Design review of the part built by this model. Coordinates are the model's own, in mm. Face numbers are marked on the shaded views. A direction names the side the tool comes from. Coordinates: 2 decimals unless noted, no trailing zeros. Loops run counter-clockwise (first coordinate to the right, second up) from the corner with the lowest first, then second, coordinate; pieces in that order, holes last. Notation, with made-up numbers: (-0.5, 78.5) - (16.5, 78.5) arc R23 cw to (16.5, 116.5) - close; hole circle Ø11 at (73, 28). An arc over 180 degrees is marked (long way). Use one line per item in the form item = value. Start each with the question number.
(1) The part is to be moulded in two halves that separate along X. For the marked faces 4, 5 and 6, say which applies: pulls with the +X half, pulls with the -X half, needs draft (parallel to the pull), parting line crosses it, or undercut.
(2) Add section A-A (z = 10.5). State the section outline as (x, y) points (1 decimal), plus the area to 3 significant figures.
(3) Clearance check with flat-ended pins moving along their axes: pin 1 Ø6 at (x, y) = (0.5, -3) entering from +Z; pin 2 Ø3 at (x, z) = (-47.5, 10.5) entering from -Y; pin 3 Ø12 at (x, y) = (34.5, 15) entering from +Z (3 decimals); pin 4 Ø16.5 at (x, y) = (2.5, -3) entering from -Z. State where each tip first meets the part, or that it passes through.
(4) For L1, parallel to Y at x = 0, z = 19.1; L2, parallel to Y at x = 0, z = 1.3; L3, parallel to Z at x = -15.5, y = 51.5 (3 decimals), list the stretches that pass through material, from the lowest coordinate up.
(5) Tool access review of the marked faces 1, 2 and 3: name each direction out of +Z, -Z, +X, -X, +Y, -Y from which nothing blocks a thin tool from reaching the whole face with its end or side.
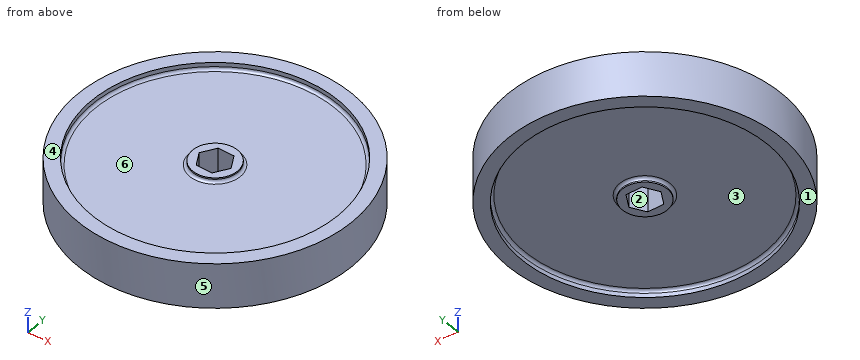
```python
from build123d import *

# Parameters (mm, degrees)
SKETCH1_R           = 61.9125
BOSS_EXTRUDE1_DEPTH = 20.32
SKETCH2_R           = 55.626
SKETCH2_R_2         = 10.16
CUT_EXTRUDE1_DEPTH  = 3.175
SKETCH3_R           = 55.626
SKETCH3_R_2         = 10.16
CUT_EXTRUDE2_DEPTH  = 3.175
SKETCH4_R           = 10.16
CUT_EXTRUDE3_DEPTH  = 1.27
SKETCH7_R           = 10.16
CUT_EXTRUDE5_DEPTH  = 1.27
FILLET1_R           = 1.27


with BuildPart() as part:
    # Sketch1 → Boss-Extrude1 (new body)
    with BuildSketch(Plane.XY):
        Circle(SKETCH1_R)
        Polygon((3.569234353, -6.4049902), (7.331501401, -0.111447478), (3.762267048, 6.293542722), (-3.569234353, 6.4049902), (-7.331501401, 0.111447478), (-3.762267048, -6.293542722), align=None, mode=Mode.SUBTRACT)
    extrude(amount=BOSS_EXTRUDE1_DEPTH)

    # Sketch2 → Cut-Extrude1 (cut)
    with BuildSketch(Plane.XY.offset(20.32)):
        Circle(SKETCH2_R)
        Circle(SKETCH2_R_2, mode=Mode.SUBTRACT)
    extrude(amount=-CUT_EXTRUDE1_DEPTH, mode=Mode.SUBTRACT)

    # Sketch3 → Cut-Extrude2 (cut)
    with BuildSketch(Plane(origin=(0, 0, 0), x_dir=(-1, 0, 0), z_dir=(0, 0, -1))):
        Circle(SKETCH3_R)
        Circle(SKETCH3_R_2, mode=Mode.SUBTRACT)
    extrude(amount=-CUT_EXTRUDE2_DEPTH, mode=Mode.SUBTRACT)

    # Sketch4 → Cut-Extrude3 (cut)
    with BuildSketch(Plane(origin=(0, 0, 0), x_dir=(-1, 0, 0), z_dir=(0, 0, -1))):
        Circle(SKETCH4_R)
    extrude(amount=-CUT_EXTRUDE3_DEPTH, mode=Mode.SUBTRACT)

    # Sketch7 → Cut-Extrude5 (cut)
    with BuildSketch(Plane.XY.offset(20.32)):
        Circle(SKETCH7_R)
    extrude(amount=-CUT_EXTRUDE5_DEPTH, mode=Mode.SUBTRACT)

    # Fillet1
    fillet1_edges = [part.edges().sort_by_distance(p)[0] for p in [
        (-55.626, 0, 17.145),
        (-10.16, 0, 17.145),
        (55.626, 0, 3.175),
        (10.16, 0, 3.175),
    ]]
    fillet(fillet1_edges, radius=FILLET1_R)


solid = part.part
```
Computed values:
q1.face_4 = needs draft
q1.face_5 = parting line crosses it
q1.face_6 = undercut
q2.outline = circle Ø123.8 at (0, 0); hole (-7.3, 0.1) - (-3.8, -6.3) - (3.6, -6.4) - (7.3, -0.1) - (3.8, 6.3) - (-3.6, 6.4) - close
q2.area = 11,900 mm^2
q3.pin_1 = through
q3.pin_2 = -41.44
q3.pin_3 = 17.145
q3.pin_4 = 1.27
q4.L1 = -61.91 to -55.63, 55.63 to 61.91
q4.L2 = -61.91 to -55.63, -10.16 to -6.35, 6.35 to 10.16, 55.63 to 61.91
q4.L3 = 3.175 to 17.145
q5.face_1 = -Z, +X, -X, +Y, -Y
q5.face_2 = +Z, -Z
q5.face_3 = -Z
